Check sheet for the modelled part. Datum: model origin and axes. Units: mm. A direction names the side the tool comes from. Coordinates: 2 decimals unless noted, no trailing zeros.
Autodesk Inventor part; units mm, degrees
ref_plane "YZ Plane" through (0, 0, 0) normal (1, 0, 0) x (0, 1, 0)
ref_plane "XZ Plane" through (0, 0, 0) normal (0, 1, 0) x (-1, 0, 0)
ref_plane "XY Plane" through (0, 0, 0) normal (0, 0, 1) x (1, 0, 0)
sketch "Skizze1" plane through (0, 0, 0) normal (0, 0, 1) x (1, 0, 0)
  line L0 (-91, 0) -> (91, 0) construction
  circle A0 centre (0, 0) radius 65
  line L1 (-6.5, 33) -> (6.5, 33)
  line L2 (6.5, 33) -> (6.5, 30)
  line L3 (6.5, 30) -> (-6.5, 30)
  line L4 (-6.5, 30) -> (-6.5, 33)
  line L5 (1.5, 30) -> (-1.5, 30)
  line L6 (-1.5, 30) -> (-1.5, 25)
  line L7 (-1.5, 25) -> (1.5, 25)
  line L8 (1.5, 25) -> (1.5, 30)
  circle A1 centre (0, 0) radius 4.5
  line L9 (0, 91) -> (0, -91) construction
  dimension "d9" = 130
  dimension "d10" = 3
  dimension "d11" = 30
  dimension "d14" = 13
  dimension "d23" = 5
  dimension "d62" = 9
extrude "Extrusion3" add sketch "Skizze1" against normal blind 7 contours L1 L2 L3 L4 | L3 L8 L7 L6
fillet "Rundung1" radius 4 2 edges at (-6.5, 31.5, -7) (6.5, 31.5, -7)
sketch "Skizze2" plane through (-6.5, 33, 0) normal (0, 1, 0) x (1, 0, 0)
  circle A0 centre (3, 4) radius 1.1
  circle A1 centre (10, 4) radius 1.1
  line L0 (6.5, 0) -> (6.5, 7) construction
  line L1 (43, 0) -> (-27, 0) construction
  line L2 (-1.6221, 4) -> (19.0112, 4) construction
  line L3 (4, 7) -> (9, 7) construction
  line L4 (0, 0) -> (0, 3)
  dimension "d16" = 2.2
  dimension "d20" = 3
  dimension "d21" = 3
extrude "Extrusion4" cut sketch "Skizze2" against normal up to next
chamfer "Fase1" distance 5 distance2 7 1 edges at (0, 25, -7) measured on face at (0.5, 32, -7)
pattern_circular "Runde Anordnung1" count 3 over 360 about axis through (0, 0, -10) along (0, 0, 1) of "Extrusion3", "Extrusion4", "Fase1", "Rundung1"
extrude "Extrusion11" add sketch "Skizze1" along normal blind 2 contours A0 | L1 L2 L3 L4 | L3 L8 L7 L6
fillet "Rundung5" radius 1 4 edges at (-65, 0, 2) (-4.5, 0, 2) (-4.5, 0, 0) (-65, 0, 0)
equation "\"d21\" = d20"
properties part number "Stewart-Plate-Head"
1) Scan lines: line 1 (Y direction, x = 0, z = 1.05); line 2 (X direction, y = 31.1, z = -4); line 3 (Z direction, x = -31, y = 31). Record each from-to range of solid material in increasing order.
Answer sheet:
line 1: y = -65 to -4.5, 4.5 to 65
line 2: x = -6.37 to -4.6, -2.4 to 2.4, 4.6 to 6.37
line 3: z = 0 to 2
2) Set-up check for faces 1 (the flat face through (-1.5, 28, -3)), 2 (the flat face through (6.5, 32, -1)), 3 (the flat face through (0, 33, -3)), 4 (the flat face through (1.5, 28, -3)), 5 (the flat face through (-23.577, -15.344, -2.673)): record each of +Z, -Z, +X, -X, +Y, -Y from which the full face is reachable in a straight line by a thin tool's end or side.
Answer sheet:
face 1: -Z, -X, -Y
face 2: -Z, +X, +Y, -Y
face 3: -Z, +X, -X, +Y
face 4: -Z, +X, -Y
face 5: -Z
3) Mould release check, pull along Z, two halves, no side actions. Record for faces 6 (the cylindrical face through (-29.91, -11.15, -5.86)), 7 (the flat face through (25.08, -12.75, -2.67)), 8 (the cylindrical face through (-25, -19, -5)), 9 (the cylindrical face through (29.453, -12.027, -4.743)): +Z half, -Z half, draft (parallel to the pull), parting line (faces both ways), or undercut.
Answer sheet:
face 6: -Z half
face 7: draft
face 8: undercut
face 9: undercut
4) Depth check by flat-ended pin: pin 1 (2.5 mm diameter, centred on y = 28.5, z = -2.5, fed in from -X); pin 2 (2.5 mm diameter, centred on y = 31.5, z = -2, fed in from -X); pin 3 (1.5 mm diameter, centred on y = 32, z = -1, fed in from +X). Enter the tip coordinate at first touch or a pass-through.
Answer sheet:
pin 1: stops at x = -1.5
pin 2: stops at x = -6.5
pin 3: stops at x = 6.5
